Part model, mm, in its own coordinate system. Face numbers are marked on the shaded views. A direction names the side the tool comes from. Give positions to 0.01 mm unless a question says otherwise; leave off trailing zeros. Write each loop counter-clockwise with the first axis right and the second up, starting at its lowest first coordinate (ties: lowest second). Pieces come first, ordered by that corner, then holes.
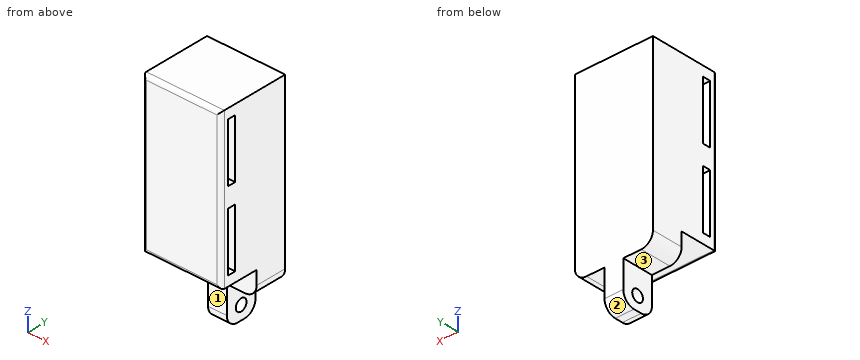
```python
from build123d import *

# Parameters (mm, degrees)
CROQUIS1_R                 = 1.5
SALIENTE_EXTRUIR1_DEPTH    = 10
CORTAR_EXTRUIR1_DEPTH      = 60.539902586
CORTAR_EXTRUIR1_DEPTH_BACK = 60.539902586
CROQUIS2_W                 = 7.6
CROQUIS2_H                 = 10
CORTAR_EXTRUIR4_DEPTH      = 60.539902586
CORTAR_EXTRUIR4_DEPTH_BACK = 60.539902586
CROQUIS4_W                 = 15
CROQUIS4_H                 = 2
REDONDEO2_R                = 1
REDONDEO3_R                = 3


with BuildPart() as part:
    # Croquis1 → Saliente-Extruir1 (new, symmetric)
    with BuildSketch(Plane(origin=(0, 0, 0), x_dir=(0, 0, -1), z_dir=(1, 0, 0))):
        Polygon((-1.5, 9), (-58, 9), (-58, -9), (-18, -9), (-18, 1), (-1.5, 1), align=None)
        with Locations((-5, 5)):
            Circle(CROQUIS1_R, mode=Mode.SUBTRACT)
    extrude(amount=SALIENTE_EXTRUIR1_DEPTH, both=True)

    # Croquis2 → Cortar-Extruir1 (cut, two sides: drawn at the far end of the back side and taken through both)
    with BuildSketch(Plane(origin=(0, 0, 0), x_dir=(1, 0, 0), z_dir=(0, 1, 0)).offset(-CORTAR_EXTRUIR1_DEPTH_BACK)):
        with Locations((-6.2, -6.5)):
            Rectangle(CROQUIS2_W, CROQUIS2_H)
        with Locations((6.2, -6.5)):
            Rectangle(CROQUIS2_W, CROQUIS2_H)
    extrude(amount=CORTAR_EXTRUIR1_DEPTH + CORTAR_EXTRUIR1_DEPTH_BACK, mode=Mode.SUBTRACT)

    # Croquis4 → Cortar-Extruir4 (cut, two sides: drawn at the far end of the back side and taken through both)
    with BuildSketch(Plane(origin=(0, 0, 0), x_dir=(0, 0, -1), z_dir=(1, 0, 0)).offset(-CORTAR_EXTRUIR4_DEPTH_BACK)):
        with Locations((-48, -6)):
            Rectangle(CROQUIS4_W, CROQUIS4_H)
        with Locations((-28, -6)):
            Rectangle(CROQUIS4_W, CROQUIS4_H)
    extrude(amount=CORTAR_EXTRUIR4_DEPTH + CORTAR_EXTRUIR4_DEPTH_BACK, mode=Mode.SUBTRACT)

    # Redondeo2
    redondeo2_edges = [part.edges().sort_by_distance(p)[0] for p in [
        (0, -9, 18),
        (0, -9, 58),
        (-10, -9, 38),
        (10, -9, 38),
    ]]
    fillet(redondeo2_edges, radius=REDONDEO2_R)

    # Redondeo3
    redondeo3_edges = [part.edges().sort_by_distance(p)[0] for p in [
        (0, 9, 1.5),
        (0, 1, 1.5),
        (-10, 5, 11.5),
        (10, 5, 11.5),
    ]]
    fillet(redondeo3_edges, radius=REDONDEO3_R)


solid = part.part
```
1) Saw through at A-A, the plane y = 5. Write the cut outline in (x, z).
Answers follow:
outline: (-10, 14.5) arc R3 ccw to (-7, 11.5) - (-2.4, 11.5) - (-2.4, 6.5) - (2.4, 6.5) - (2.4, 11.5) - (7, 11.5) arc R3 ccw to (10, 14.5) - (10, 58) - (-10, 58) - close; (-2.4, 1.5) - (2.4, 1.5) - (2.4, 3.5) - (-2.4, 3.5) - close
2) Saw through at B-B, the plane x = -3.75. Write the cut outline in (y, z), then the cut area to 3 significant figures.
Answers follow:
outline: (-9, 19) arc R1 ccw to (-8, 18) - (1, 18) - (1, 11.5) - (9, 11.5) - (9, 58) - (-8, 58) arc R1 ccw to (-9, 57) - close; hole (-7, 20.5) - (-5, 20.5) - (-5, 35.5) - (-7, 35.5) - close; hole (-7, 40.5) - (-5, 40.5) - (-5, 55.5) - (-7, 55.5) - close
area: 712 mm2
3) Saw through at D-D, the plane x = 0.75. Write the cut outline in (y, z).
Answers follow:
outline: (-9, 19) arc R1 ccw to (-8, 18) - (1, 18) - (1, 4.5) arc R3 ccw to (4, 1.5) - (6, 1.5) arc R3 ccw to (9, 4.5) - (9, 58) - (-8, 58) arc R1 ccw to (-9, 57) - close; hole (-7, 20.5) - (-5, 20.5) - (-5, 35.5) - (-7, 35.5) - close; hole (-7, 40.5) - (-5, 40.5) - (-5, 55.5) - (-7, 55.5) - close; hole circle Ø3 at (5, 5)
4) Saw through at C-C, the plane z = 53.5. Write the cut outline in (x, y), then the cut area to 3 significant figures.
Answers follow:
outline: (-10, -8) arc R1 ccw to (-9, -9) - (9, -9) arc R1 ccw to (10, -8) - (10, -7) - (-10, -7) - close; (-10, -5) - (10, -5) - (10, 9) - (-10, 9) - close
area: 320 mm2
5) Pin check, flat tips, straight feed: pin 1 Ø8 at (x, y) = (-4.5, -7) entering from -Z; pin 2 Ø4 at (y, z) = (5, 5) entering from +X; pin 3 Ø1.4 at (x, y) = (-4.5, 5.5) entering from -Z. Stop position of each tip, or through.
Answers follow:
pin 1: stops at z = 18
pin 2: stops at x = 2.4
pin 3: stops at z = 11.5
6) Wall check: L1, parallel to Z at x = -1.05, y = 5; L2, parallel to Y at x = -4, z = 43; L3, parallel to Y at x = -0.45, z = 5. Give the ranges that are in metal, low to high.
Answers follow:
L1: z = 1.5 to 3.5, 6.5 to 58
L2: y = -9 to -7, -5 to 9
L3: y = 1 to 3.5, 6.5 to 9
7) 3-axis set-ups, long thin cutter, end or side, ignore diameter. For the marked faces 1, 2 and 3: which of +Z, -Z, +X, -X, +Y, -Y reach the whole face in a straight line?
Answers follow:
face 1: -Z, +X, -X, -Y
face 2: -Z, +X, -X, +Y
face 3: -Z, -X, +Y, -Y
